The listing builds one solid part. Answer for the finished solid, in the listing's coordinates (mm). Give positions to 0.01 mm unless a question says otherwise; leave off trailing zeros. Loops run counter-clockwise (first coordinate to the right, second up) from the corner with the lowest first, then second, coordinate; pieces in that order, holes last.
Item 1: Each of these flat-tipped pins is pushed along its axis until it touches: pin 1 Ø3 at (x, y) = (-1, 20) entering from +Z; pin 2 Ø4.5 at (x, y) = (-2, 17) entering from -Z; pin 3 Ø12 at (y, z) = (19, 5) entering from -X; pin 4 Ø2.5 at (x, y) = (0.5, 19.99) entering from +Z. Where does it stop, or does it pass through?
Item 2: The mould has two halves that part along Y. Classify faces 1 (the face through (-0.61, 21.01, -0.03)), 2 (the face through (0.72, 24.99, -0.03)), 3 (the face through (3, -5, 15)): pulls with the +Y half, pulls with the -Y half, needs draft (parallel to the pull), parting line crosses it, or undercut.
Item 3: Section C-C, the plane z = 2.75 is taken. Give the vertices of the cut face in (x, y), and give its area (3 significant figures).
Item 4: Section A-A, the plane x = -2.75 is taken. Give the vertices of the cut face in (y, z).
Item 5: Consider line 1 along Y through (x, z) = (0, -7.5); line 2 along Z through (x, y) = (1.75, 15.5); line 3 along Y through (x, z) = (-4.75, 4). Determine where each line is inside the solid, lowest interval first.
Item 6: Section B-B, the plane x = 0 is taken. Give the vertices of the cut face in (y, z).
Item 7: Section D-D, the plane y = 7 is taken. Give the vertices of the cut face in (x, z).
from build123d import *

# Parameters (mm, degrees)
BOSS_EXTRU_2_DEPTH      = 2
BOSS_EXTRU_2_DEPTH_BACK = 2
ESQUISSE1_R             = 5.3
ESQUISSE1_R_2           = 1.5
ESQUISSE2_R             = 7.5
ESQUISSE2_R_2           = 5.3
BOSS_EXTRU_3_DEPTH      = 13


with BuildPart() as part:
    # Esquisse1 → Boss.-Extru.2 (new, two sides: drawn at the far end of the back side and taken through both)
    with BuildSketch(Plane.XY.offset(-BOSS_EXTRU_2_DEPTH_BACK)):
        with BuildLine():
            ThreePointArc((-7.5, 0), (0, -7.5), (7.5, 0))
            Line((7.5, 0), (5.471395589, 20.4865521))
            ThreePointArc((5.471395589, 20.4865521), (0.614199015, 24.992451663), (-4.451008104, 20.721717969))
            Line((-4.451008104, 20.721717969), (-7.5, 0))
        make_face()
        Circle(ESQUISSE1_R, mode=Mode.SUBTRACT)
        with Locations((0.495729813, 19.993855355)):
            Circle(ESQUISSE1_R_2, mode=Mode.SUBTRACT)
    extrude(amount=BOSS_EXTRU_2_DEPTH + BOSS_EXTRU_2_DEPTH_BACK)

    # Esquisse2 → Boss.-Extru.3 (add)
    with BuildSketch(Plane.XY.offset(2)):
        Circle(ESQUISSE2_R)
        Circle(ESQUISSE2_R_2, mode=Mode.SUBTRACT)
    boss_extru_3 = extrude(amount=BOSS_EXTRU_3_DEPTH)

    # Symétrie1: Boss.-Extru.3 across plane
    add(boss_extru_3.mirror(Plane.XY))


solid = part.part
Worked answers:
1. pin 1: stops at z = 2
1. pin 2: stops at z = -2
1. pin 3: stops at x = -5.47
1. pin 4: passes through
2. face 1: undercut
2. face 2: pulls with the +Y half
2. face 3: needs draft
3. outline: circle Ø15 at (0, 0); hole circle Ø10.6 at (0, 0)
3. area: 88.5 mm2
4. outline: (-6.98, -15) - (-4.53, -15) - (-4.53, 15) - (-6.98, 15) - close; (4.53, -15) - (6.98, -15) - (6.98, -2) - (23.8, -2) - (23.8, 2) - (6.98, 2) - (6.98, 15) - (4.53, 15) - close
5. line 1: y = -7.5 to -5.3, 5.3 to 7.5
5. line 2: z = -2 to 2
5. line 3: y = -5.8 to -2.35, 2.35 to 5.8
6. outline: (-7.5, -15) - (-5.3, -15) - (-5.3, 15) - (-7.5, 15) - close; (5.3, -15) - (7.5, -15) - (7.5, -2) - (18.58, -2) - (18.58, 2) - (7.5, 2) - (7.5, 15) - (5.3, 15) - close; (21.41, -2) - (24.97, -2) - (24.97, 2) - (21.41, 2) - close
7. outline: (-6.47, -2) - (-2.69, -2) - (-2.69, -15) - (2.69, -15) - (2.69, -2) - (6.81, -2) - (6.81, 2) - (2.69, 2) - (2.69, 15) - (-2.69, 15) - (-2.69, 2) - (-6.47, 2) - close
